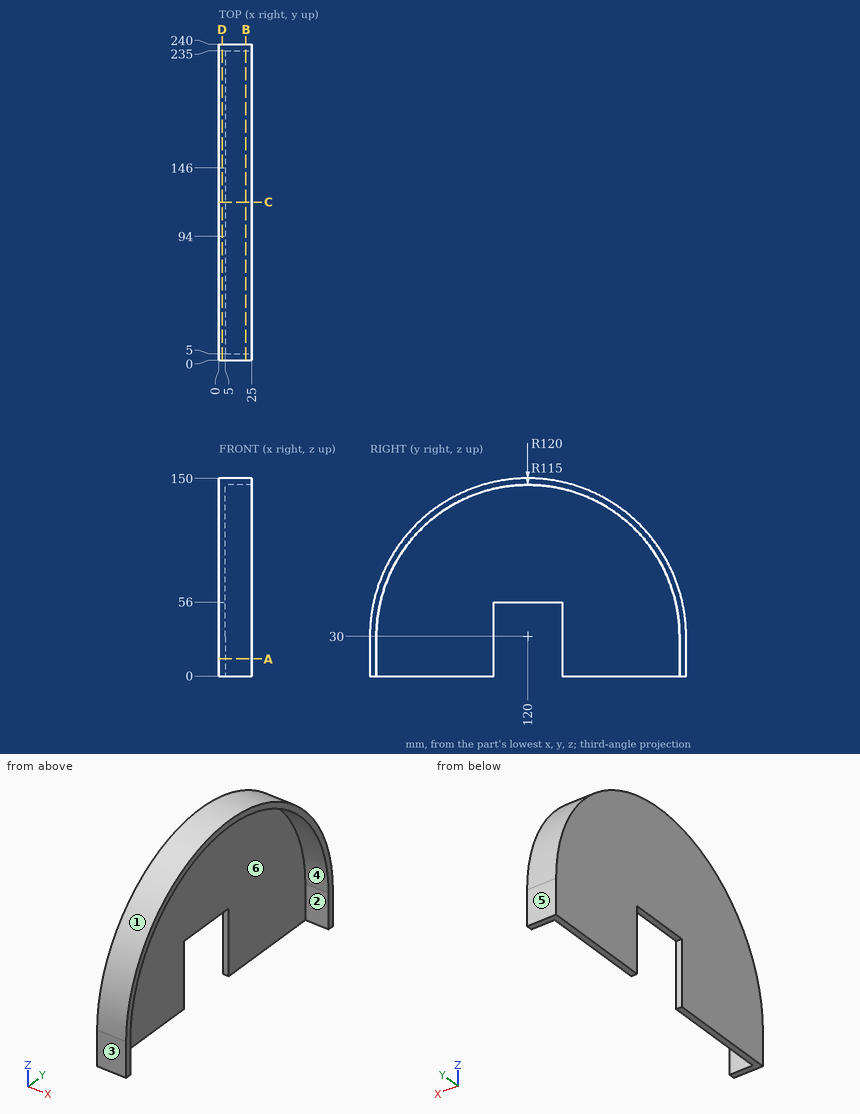
Verification items for this drawing (mm, ordinates from the low corner). A direction names the side the tool comes from. Coordinates: 2 decimals unless noted, no trailing zeros. Loops run counter-clockwise (first coordinate to the right, second up) from the corner with the lowest first, then second, coordinate; pieces in that order, holes last.
Item 1: Sectioned sample at D-D, the plane x = 2.5. Record the boundary of the cut face in (y, z), then the cut area to 3 significant figures.
Item 2: Sectioned sample at A-A, the plane z = 13. Record the boundary of the cut face in (x, y).
Item 3: Go/stop test with flat-tipped pins: pin 1 Ø1.5 at (x, z) = (9, 64.5) entering from -Y; pin 2 Ø8 at (x, y) = (13, 110) entering from -Z; pin 3 Ø2.5 at (x, y) = (3, 121) entering from -Z. Record where each tip stops, or that it passes through.
Item 4: Sectioned sample at C-C, the plane y = 120. Record the boundary of the cut face in (x, z), then the cut area to 3 significant figures.
Item 5: Access from +Z, -Z, +X, -X, +Y, -Y to the whole of each face (thin tool, end or side, straight path). Record for the marked faces 1 and 2.
Item 6: Thickness scan on line 1 (Y direction, x = 8, z = 8); line 2 (X direction, y = 200, z = 32.5); line 3 (Y direction, x = 10.25, z = 64.5). Record the ranges inside material, lowest first.
Item 7: Release check for a two-part mould opening along Y. For the marked faces 3, 4, 5 and 6 record: released by +Y, released by -Y, zero draft, split by the parting line, or undercut.
Item 8: Sectioned sample at B-B, the plane x = 20.5. Record the boundary of the cut face in (y, z), then the cut area to 3 significant figures.
Check result:
1. outline: (0, 0) - (94, 0) - (94, 56) - (146, 56) - (146, 0) - (240, 0) - (240, 30) arc R120 ccw to (0, 30) - close
1. area: 26,900 mm2
2. outline: (0, 0) - (25, 0) - (25, 5) - (5, 5) - (5, 94) - (0, 94) - close; (0, 146) - (5, 146) - (5, 235) - (25, 235) - (25, 240) - (0, 240) - close
3. pin 1: stops at y = 4.84
3. pin 2: stops at z = 144.14
3. pin 3: stops at z = 56
4. outline: (0, 56) - (5, 56) - (5, 145) - (25, 145) - (25, 150) - (0, 150) - close
4. area: 570 mm2
5. face 1: +Z, +X, -X
5. face 2: -Z, +X
6. line 1: y = 0 to 5, 235 to 240
6. line 2: x = 0 to 5
6. line 3: y = 5.07 to 10.3, 229.7 to 234.93
7. face 3: released by -Y
7. face 4: undercut
7. face 5: released by +Y
7. face 6: undercut
8. outline: (0, 0) - (5, 0) - (5, 30) arc R115 cw to (235, 30) - (235, 0) - (240, 0) - (240, 30) arc R120 ccw to (0, 30) - close
8. area: 2,150 mm2
